Part model, mm, in its own coordinate system. Face numbers are marked on the shaded views. A direction names the side the tool comes from. Round coordinates to 2 decimals unless told otherwise and drop trailing zeros. Write each loop counter-clockwise with the first axis right and the second up, starting at its lowest first coordinate (ties: lowest second). Pieces come first, ordered by that corner, then holes. Notation, with made-up numbers: M 13,84.25 L 42,84.25 A17 ccw 42,104.25 Z; hole C 7.25,80.25 d9. An arc over 180 degrees is marked long. Use a Markdown table: item, result. Add a question column.
1) Slice it at A-A on z = 0. Give the number of separate pieces and of enclosed holes in the cut face, plus the area to 3 significant figures.
2) Two-plate mould, pull along Z, no slides. Class the marked faces 4, 5, 6 and 7: released by +Z, released by -Z, zero draft, split by the parting line, or undercut.
3) Slice it at B-B on y = 33.5. Write the cut outline in (x, z).
4) Wall check: probe 1 along X at (y, z) = (5.5, -2.25); probe 2 along X at (y, z) = (63.9, 0); probe 3 along Z at (x, y) = (61.4, 51). Give the ranges that are in metal, low to high.
5) Slice it at C-C on x = 75.8. Write the cut outline in (y, z).
6) Which spindle directions (+Z, -Z, +X, -X, +Y, -Y) get a long thin tool onto all of the face, cutting with end or side? Do the marked faces 1, 2 and 3. Say none if no direction does.
7) Drop flat-ended pins along their axis: P1, Ø5, axis at x = 64.5, y = 54, coming from the +Z side; P2, Ø8, axis at y = 11.5, z = 5.5, coming from the +X side; P3, Ø4.5, axis at y = 44, z = -10, coming from the -X side; P4, Ø14.5, axis at x = -28.5, z = 3, coming from the +Y side. Give the stop position or say it passes through.
8) Slice it at D-D on z = -11. Write the cut outline in (x, y), plus the area to 3 significant figures.
```python
from build123d import *

# Parameters (mm, degrees)
SKETCH1_W           = 125
SKETCH1_H           = 25.4
BOSS_EXTRUDE1_DEPTH = 5
SKETCH2_W           = 119
SKETCH2_H           = 17.4
CUT_EXTRUDE1_DEPTH  = 2
FILLET1_R           = 5
SKETCH3_W           = 3
SKETCH3_H           = 25.4
BOSS_EXTRUDE2_DEPTH = 60
CHAMFER1_SIZE       = 2
SKETCH4_R           = 6
CUT_EXTRUDE3_DEPTH  = 135.4
SKETCH5_W           = 25.4
SKETCH5_H           = 3
BOSS_EXTRUDE3_DEPTH = 24
SKETCH6_W           = 25.4
SKETCH6_H           = 3
BOSS_EXTRUDE4_DEPTH = 24
SKETCH9_R           = 1.75
CUT_EXTRUDE4_DEPTH  = 4
CHAMFER2_SIZE       = 7
BOSS_EXTRUDE5_DEPTH = 4
BOSS_EXTRUDE6_DEPTH = 4
CHAMFER3_SIZE       = 2
CHAMFER4_SIZE       = 3
FILLET5_R           = 2
FILLET6_R           = 3


# Some blends are built 0.0001 mm under size
with BuildPart() as part:
    # Sketch1 → Boss-Extrude1 (new body)
    with BuildSketch(Plane(origin=(0, 0, 0), x_dir=(1, 0, 0), z_dir=(0, 1, 0))):
        Rectangle(SKETCH1_W, SKETCH1_H)
    extrude(amount=BOSS_EXTRUDE1_DEPTH)

    # Sketch2 → Cut-Extrude1 (cut)
    with BuildSketch(Plane(origin=(0, 5, 0), x_dir=(1, 0, 0), z_dir=(0, 1, 0))):
        Rectangle(SKETCH2_W, SKETCH2_H)
    extrude(amount=-CUT_EXTRUDE1_DEPTH, mode=Mode.SUBTRACT)

    # Fillet1
    fillet1_edges = [part.edges().sort_by_distance(p)[0] for p in [
        (59.5, 4, -8.7),
        (59.5, 4, 8.7),
        (-59.5, 4, 8.7),
        (-59.5, 4, -8.7),
    ]]
    fillet(fillet1_edges, radius=FILLET1_R)

    # Sketch3 → Boss-Extrude2 (add)
    with BuildSketch(Plane(origin=(0, 5, 0), x_dir=(1, 0, 0), z_dir=(0, 1, 0))):
        with Locations((61, 0)):
            Rectangle(SKETCH3_W, SKETCH3_H)
        with Locations((-61, 0)):
            Rectangle(SKETCH3_W, SKETCH3_H)
    extrude(amount=BOSS_EXTRUDE2_DEPTH)

    # Chamfer1
    chamfer1_edges = [part.edges().sort_by_distance(p)[0] for p in [
        (-62.5, 0, 0),
        (62.5, 0, 0),
    ]]
    chamfer(chamfer1_edges, length=CHAMFER1_SIZE)

    # Sketch4 → Cut-Extrude3 (cut)
    with BuildSketch(Plane(origin=(62.5, 0, 0), x_dir=(0, 0, -1), z_dir=(1, 0, 0))):
        with Locations((0, 51)):
            Circle(SKETCH4_R)
    extrude(amount=-CUT_EXTRUDE3_DEPTH, mode=Mode.SUBTRACT)

    # Sketch5 → Boss-Extrude3 (add)
    with BuildSketch(Plane.ZY.offset(62.5)):
        with Locations((0, 63.5)):
            Rectangle(SKETCH5_W, SKETCH5_H)
    extrude(amount=BOSS_EXTRUDE3_DEPTH)

    # Sketch6 → Boss-Extrude4 (add)
    with BuildSketch(Plane(origin=(62.5, 0, 0), x_dir=(0, 0, -1), z_dir=(1, 0, 0))):
        with Locations((0, 63.5)):
            Rectangle(SKETCH6_W, SKETCH6_H)
    extrude(amount=BOSS_EXTRUDE4_DEPTH)

    # Sketch9 → Cut-Extrude4 (cut)
    with BuildSketch(Plane(origin=(0, 65, 0), x_dir=(1, 0, 0), z_dir=(0, 1, 0))):
        with Locations(Location((75.8, 0, 0), (0, 0, 270))):
            Circle(SKETCH9_R)
        with Locations(Location((-75.8, 0, 0), (0, 0, 270))):
            Circle(SKETCH9_R)
    extrude(amount=-CUT_EXTRUDE4_DEPTH, mode=Mode.SUBTRACT)

    # Chamfer2
    chamfer2_edges = [part.edges().sort_by_distance(p)[0] for p in [
        (-86.5, 63.5, -12.7),
        (-86.5, 63.5, 12.7),
        (86.5, 63.5, 12.7),
        (86.5, 63.5, -12.7),
    ]]
    chamfer(chamfer2_edges, length=CHAMFER2_SIZE)

    # Sketch10 → Boss-Extrude5 (add)
    with BuildSketch(Plane.XY.offset(12.7)):
        Polygon((-69.5, 65), (-64.924872653, 69.5), (-55, 69.5), (-55, 5), (-59.5, 5), (-59.5, 65), align=None)
        Polygon((69.5, 65), (65.073893694, 69.5), (55, 69.5), (55, 5), (59.5, 5), (59.5, 65), align=None)
    extrude(amount=-BOSS_EXTRUDE5_DEPTH)

    # Sketch11 → Boss-Extrude6 (add)
    with BuildSketch(Plane(origin=(0, 0, -12.7), x_dir=(-1, 0, 0), z_dir=(0, 0, -1))):
        Polygon((-69.5, 65), (-65.073893694, 69.5), (-55, 69.5), (-55, 5), (-59.5, 5), (-59.5, 65), align=None)
        Polygon((69.5, 65), (64.924872653, 69.5), (55, 69.5), (55, 5), (59.5, 5), (59.5, 65), align=None)
    extrude(amount=-BOSS_EXTRUDE6_DEPTH)

    # Chamfer3
    chamfer3_edges = [part.edges().sort_by_distance(p)[0] for p in [
        (-55, 69.5, 10.7),
        (55, 69.5, 10.7),
        (55, 69.5, -10.7),
        (-55, 69.5, -10.7),
    ]]
    chamfer(chamfer3_edges, length=CHAMFER3_SIZE)

    # Chamfer4
    # the kernel refuses this chamfer: 3 mm, written as the material it adds along each edge
    with BuildSketch(Plane(origin=(-55, 5, 12.7), x_dir=(-0.02749587661058672, 0.9996219169112968, 0), z_dir=(0, 0, -1)), Plane(origin=(55, 5, 12.7), x_dir=(-0.9996219169112968, -0.02749587661058648, 0), z_dir=(0, 0, -1)), Plane(origin=(-55, 5, -12.7), x_dir=(0.9996219169112968, -0.02749587661058648, 0), z_dir=(0, 0, 1))) as chamfer4_piece_1:
        Polygon((CHAMFER4_SIZE * 0.999621916911, CHAMFER4_SIZE * 0.0274958766106), (-CHAMFER4_SIZE * 0.0274958766106, CHAMFER4_SIZE * 0.999621916911), (0, 0), align=None)
    extrude(amount=4)
    with BuildSketch(Plane(origin=(55, 5, -12.7), x_dir=(-0.9996219169112968, -0.02749587661058648, 0), z_dir=(0, 0, 1))) as chamfer4_piece_2:
        Polygon((CHAMFER4_SIZE * 0.999621916911, -CHAMFER4_SIZE * 0.0274958766106), (-CHAMFER4_SIZE * 0.0274958766106, -CHAMFER4_SIZE * 0.999621916911), (0, 0), align=None)
    extrude(amount=4)

    # Fillet5
    fillet5_edges = [part.edges().sort_by_distance(p)[0] for p in [
        (-58.035533906, 3, 7.235533906),
        (-59.5, 3, 0),
        (-58.035533906, 3, -7.235533906),
        (0, 3, -8.7),
        (58.035533906, 3, -7.235533906),
        (59.5, 3, 0),
        (58.035533906, 3, 7.235533906),
        (0, 3, 8.7),
    ]]
    fillet(fillet5_edges, radius=FILLET5_R - 0.0001)  # a hair under: the kernel refuses the full size

    # Fillet6
    fillet6_edges = [part.edges().sort_by_distance(p)[0] for p in [
        (-64.5, 65, 8.7),
        (-59.5, 35, 8.7),
        (64.5, 65, 8.7),
        (59.5, 35, 8.7),
        (64.5, 65, -8.7),
        (59.5, 35, -8.7),
        (-64.5, 65, -8.7),
        (-59.5, 35, -8.7),
    ]]
    fillet(fillet6_edges, radius=FILLET6_R)


solid = part.part
```
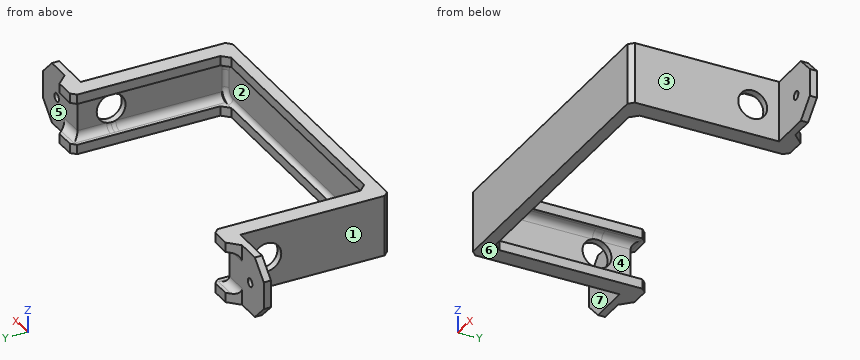
Entries:
| question | item | result |
|---|---|---|
| 1 | separate pieces | 5 |
| 1 | enclosed holes | 0 |
| 1 | area | 796 mm^2 |
| 2 | face 4 | undercut |
| 2 | face 5 | undercut |
| 2 | face 6 | released by -Z |
| 2 | face 7 | zero draft |
| 3 | outline | M -62.5,-12.7 L -55,-12.7 L -55,-8.7 L -56.5,-8.7 A3 cw -59.5,-5.7 L -59.5,5.7 A3 cw -56.5,8.7 L -55,8.7 L -55,12.7 L -62.5,12.7 Z; M 55,-12.7 L 62.5,-12.7 L 62.5,12.7 L 55,12.7 L 55,8.7 L 56.5,8.7 A3 cw 59.5,5.7 L 59.5,-5.7 A3 cw 56.5,-8.7 L 55,-8.7 Z |
| 4 | probe 1 | x = -62.5 to -59.5, 59.5 to 62.5 |
| 4 | probe 2 | x = -86.5 to -77.55, -74.05 to -59.5, 59.5 to 74.05, 77.55 to 86.5 |
| 4 | probe 3 | z = -12.7 to -6, 6 to 12.7 |
| 5 | outline | M 62,-12.7 L 65,-12.7 L 65,-1.75 L 62,-1.75 Z; M 62,1.75 L 65,1.75 L 65,12.7 L 62,12.7 Z |
| 6 | face 1 | +Z, -Z, -X, -Y |
| 6 | face 2 | +Y |
| 6 | face 3 | +Z, -Z, +X, -Y |
| 7 | P1 | stops at z = 12.7 |
| 7 | P2 | stops at x = 62.5 |
| 7 | P3 | stops at x = -62.5 |
| 7 | P4 | stops at y = 5 |
| 8 | outline | M -81.2,62 L -62.5,62 L -62.5,2 L -60.5,0 L 60.5,0 L 62.5,2 L 62.5,62 L 81.2,62 L 81.2,65 L 69.5,65 L 65.07,69.5 L 57,69.5 L 55,67.5 L 55,8 L 52,5 L -52,5 L -55,8 L -55,67.5 L -57,69.5 L -64.92,69.5 L -69.5,65 L -81.2,65 Z |
| 8 | area | 1,750 mm^2 |
